```python
from build123d import *

# Parameters (mm, degrees)
F0_W     = 50.8
F0_H     = 25.4
F0_W_2   = 47.625
F0_H_2   = 22.225
F1_DEPTH = 3.175
F2_W     = 46.99
F2_H     = 21.59
F3_DEPTH = 3.175
F4_W     = 43.18
F4_H     = 17.78
F5_DEPTH = 3.175
F6_R     = 2.54


with BuildPart() as f1:
    # F0 (on Front) → F1 (new body)
    with BuildSketch(Plane.XZ):
        Rectangle(F0_W, F0_H)
        Rectangle(F0_W_2, F0_H_2, mode=Mode.SUBTRACT)
        Rectangle(F0_W_2, F0_H_2)
    extrude(amount=F1_DEPTH)

    # F2 (on face) → F3 (join)
    with BuildSketch(Plane.XZ.offset(3.175)):
        Rectangle(F2_W, F2_H)
    extrude(amount=F3_DEPTH)

    # F4 (on face) → F5 (cut)
    with BuildSketch(Plane.XZ.offset(6.35)):
        Rectangle(F4_W, F4_H)
    extrude(amount=-F5_DEPTH, mode=Mode.SUBTRACT)

    # F6
    f6_edges = [f1.edges().sort_by_distance(p)[0] for p in [
        (-25.4, -1.5875, -12.7),
        (25.4, -1.5875, -12.7),
        (25.4, -1.5875, 12.7),
        (-25.4, -1.5875, 12.7),
    ]]
    fillet(f6_edges, radius=F6_R)


solid = f1.part
```
The listing builds one solid part. Answer for the finished solid, in the listing's coordinates (mm). A direction names the side the tool comes from. Coordinates: 2 decimals unless noted, no trailing zeros. Write each loop counter-clockwise with the first axis right and the second up, starting at its lowest first coordinate (ties: lowest second). Pieces come first, ordered by that corner, then holes. Notation, with made-up numbers: (80.5, 8) - (106.5, 8) arc R20 ccw to (106.5, 30) - close; hole circle Ø9 at (-31, 17). An arc over 180 degrees is marked (long way). One line per item, written item: value.
1) A tool of negligible diameter and unlimited length cuts with its end or side. For faces 4 (the flat face through (21.59, -5, 0)), 5 (the flat face through (0, -5, 10.795)), 6 (the flat face through (0, -5, -10.795)), 7 (the flat face through (23.495, -5, 0)), 8 (the flat face through (-23.495, -5, 0)), from which of +Z, -Z, +X, -X, +Y, -Y can it reach the whole face along a straight path? Write none if from no direction.
Geometry check:
face 4: -Y
face 5: +Z, +X, -X, -Y
face 6: -Z, +X, -X, -Y
face 7: +Z, -Z, +X, -Y
face 8: +Z, -Z, -X, -Y
2) Each of these flat-tipped pins is pushed along its axis until it touches: pin 1 Ø4 at (x, z) = (20, -0.5) entering from -Y; pin 2 Ø1 at (y, z) = (-4, 3) entering from +X (3 decimals); pin 3 Ø2.5 at (x, y) = (7.5, -5) entering from -Z (3 decimals); pin 4 Ø1 at (x, z) = (3.5, -2.5) entering from -Y (3 decimals). Where does it stop, or does it pass through?
Geometry check:
pin 1: stops at y = -6.35
pin 2: stops at x = 23.495
pin 3: stops at z = -10.795
pin 4: stops at y = -3.175
3) Find section B-B (z = 5). Give the vertices of the cut face in (x, y) (3 decimals).
Geometry check:
outline: (-25.4, -3.175) - (-23.495, -3.175) - (-23.495, -6.35) - (-21.59, -6.35) - (-21.59, -3.175) - (21.59, -3.175) - (21.59, -6.35) - (23.495, -6.35) - (23.495, -3.175) - (25.4, -3.175) - (25.4, 0) - (-25.4, 0) - close
4) Consider line 1 along X through (y, z) = (-3.25, -7) (3 decimals); line 2 along Z through (x, y) = (5.5, -4.25) (3 decimals); line 3 along Y through (x, z) = (14, 11.25) (3 decimals). Determine where each line is inside the solid, lowest interval first. Write a range as from..to.
Geometry check:
line 1: x = -23.495..-21.59, 21.59..23.495
line 2: z = -10.795..-8.89, 8.89..10.795
line 3: y = -3.175..0
5) For a pull along X with two mould halves and no side action, classify faces 1 (the cylindrical face through (24.636, -1.61, -11.976)), 2 (the flat face through (0, -3.175, -11)), 3 (the flat face through (-21.59, -5, 0)) as pulls with the +X half, pulls with the -X half, needs draft (parallel to the pull), parting line crosses it, or undercut.
Geometry check:
face 1: pulls with the +X half
face 2: needs draft
face 3: undercut
6) Find section C-C (x = 16.5). Give the vertices of the cut face in (y, z) (3 decimals), and give its area (3 significant figures).
Geometry check:
outline: (-6.35, -10.795) - (-3.175, -10.795) - (-3.175, -12.7) - (0, -12.7) - (0, 12.7) - (-3.175, 12.7) - (-3.175, 10.795) - (-6.35, 10.795) - (-6.35, 8.89) - (-3.175, 8.89) - (-3.175, -8.89) - (-6.35, -8.89) - close
area: 92.7 mm2
7) Find section A-A (y = -4.5). Give the vertices of the cut face in (x, z) (3 decimals).
Geometry check:
outline: (-23.495, -10.795) - (23.495, -10.795) - (23.495, 10.795) - (-23.495, 10.795) - close; hole (-21.59, -8.89) - (21.59, -8.89) - (21.59, 8.89) - (-21.59, 8.89) - close
